```python
from build123d import *

# Parameters (mm, degrees)
F1_DEPTH  = 45
F2_R      = 6
F3_DEPTH  = 10.001
F6_DEPTH  = 6
F7_R      = 10
F8_DEPTH  = 37.5
F10_DEPTH = 3


# Not quite as in the source:
# - a pattern or mirror of a feature is missing from the dataset's text; its kind, count and spacing are read off the source's solid


with BuildPart() as f1:
    # F0 (on Right) → F1 (new body, symmetric)
    with BuildSketch(Plane.YZ):
        Polygon((27.5, -20), (77.5, -20), (77.5, -10), (37.5, -10), (37.5, 0), (-37.5, 0), (-37.5, -10), (-77.5, -10), (-77.5, -20), (-27.5, -20), (-27.5, -10), (27.5, -10), align=None)
    extrude(amount=F1_DEPTH, both=True)

    # F2 (on face) → F3 (cut, through all)
    with BuildSketch(Plane.XY.offset(-10)):
        with Locations((25, -52.5)):
            Circle(F2_R)
        with Locations((-25, -52.5)):
            Circle(F2_R)
        with Locations((-25, 52.5)):
            Circle(F2_R)
        with Locations((25, 52.5)):
            Circle(F2_R)
    extrude(amount=-F3_DEPTH, mode=Mode.SUBTRACT)

    # F5 (on offset) → F6 (join)
    with BuildSketch(Plane(origin=(-8, 0, 0), x_dir=(0, -1, 0), z_dir=(-1, 0, 0))):
        Polygon((-37.5, -10), (-37.5, 0), (-77.5, -10), align=None)
    f6 = extrude(amount=-F6_DEPTH)

    # F6_copies: F6 across plane
    add(f6.mirror(Plane(origin=(0, 0, 0), x_dir=(0, 0, -1), z_dir=(0, -1, 0))))

    # F7 (on Front) → F8 (join, symmetric)
    with BuildSketch(Plane.XZ):
        with BuildLine():
            Line((5, 0), (45, 0))
            Line((45, 0), (45, 35))
            ThreePointArc((45, 35), (25, 55), (5, 35))
            Line((5, 35), (5, 0))
        make_face()
        with Locations((25, 35)):
            Circle(F7_R, mode=Mode.SUBTRACT)
    extrude(amount=F8_DEPTH, both=True)

    # F9 (on Front) → F10 (join, symmetric)
    with BuildSketch(Plane.XZ):
        Polygon((11.7812880283, 50.0088525148), (-45, 0), (5, 0), align=None)
    extrude(amount=F10_DEPTH, both=True)


solid = f1.part
```
Read the model definition and answer for the solid it produces. Units are mm, in the model's axes. A direction names the side the tool comes from. Coordinates: 2 decimals unless noted, no trailing zeros. Loops run counter-clockwise (first coordinate to the right, second up) from the corner with the lowest first, then second, coordinate; pieces in that order, holes last. Notation, with made-up numbers: (73, 39.25) - (115, 39.25) arc R24 ccw to (115, 50.25) - close; hole circle Ø7 at (54, -32.75). An arc over 180 degrees is marked (long way). Answer in a Markdown table with one row per item.
1. Find section C-C, the plane x = 22. Write down the section's boundary in (y, z), then the cut area to 3 significant figures.
Conclusion:
| item | result |
|---|---|
| outline | (-77.5, -20) - (-57.7, -20) - (-57.7, -10) - (-77.5, -10) - close; (-47.3, -20) - (-27.5, -20) - (-27.5, -10) - (27.5, -10) - (27.5, -20) - (47.3, -20) - (47.3, -10) - (37.5, -10) - (37.5, 25.46) - (-37.5, 25.46) - (-37.5, -10) - (-47.3, -10) - close; (-37.5, 44.54) - (37.5, 44.54) - (37.5, 54.77) - (-37.5, 54.77) - close; (57.7, -20) - (77.5, -20) - (77.5, -10) - (57.7, -10) - close |
| area | 4,220 mm² |
2. Find section A-A, the plane z = 38. Write down the section's boundary in (x, y), then the cut area to 3 significant figures.
Conclusion:
| item | result |
|---|---|
| outline | (-1.85, -3) - (5.23, -3) - (5.23, -37.5) - (15.46, -37.5) - (15.46, 37.5) - (5.23, 37.5) - (5.23, 3) - (-1.85, 3) - close; (34.54, -37.5) - (44.77, -37.5) - (44.77, 37.5) - (34.54, 37.5) - close |
| area | 1,580 mm² |
3. Given pin 1 (5 mm diameter, centred on x = 33.5, z = 41, fed in from -Y); pin 2 (10.5 mm diameter, centred on y = -21, z = 16.5, fed in from -X); pin 3 (17 mm diameter, centred on x = -27.5, y = 27, fed in from +Z), each flat-ended and moving along its own axis, determine where each tip first touches the part or whether it passes through.
Conclusion:
| item | result |
|---|---|
| pin 1 | stops at y = -37.5 |
| pin 2 | stops at x = 5 |
| pin 3 | stops at z = 0 |
4. Determine the mould class of faces 4 (the face through (-29.76, 48.85, -14.93)), 5 (the face through (-26, -37.5, -5)), 6 (the face through (-2, -49, -7)) for opening direction Y: +Y half, -Y half, draft (parallel to the pull), parting line (faces both ways), or undercut.
Conclusion:
| item | result |
|---|---|
| face 4 | undercut |
| face 5 | -Y half |
| face 6 | draft |
5. Find section B-B, the plane y = 52.5. Write down the section's boundary in (x, z), then the cut area to 4 significant figures.
Conclusion:
| item | result |
|---|---|
| outline | (-45, -20) - (-31, -20) - (-31, -10) - (-45, -10) - close; (-19, -20) - (19, -20) - (19, -10) - (-2, -10) - (-2, -3.75) - (-8, -3.75) - (-8, -10) - (-19, -10) - close; (31, -20) - (45, -20) - (45, -10) - (31, -10) - close |
| area | 697.5 mm² |
6. Which of the six approach directions +Z, -Z, +X, -X, +Y, -Y give full straight-line access (tool end or side, diameter ignored) to faces 1 (the face through (-20, -20, 0)), 2 (the face through (-8, 49, -7)), 3 (the face through (1, -27.5, -15))?
Conclusion:
| item | result |
|---|---|
| face 1 | +Z, -X, -Y |
| face 2 | +Z, -X, +Y |
| face 3 | -Z, +X, -X |
7. Straight lines are drawn through the part: line 1 (X direction, y = 52, z = -14); line 2 (Y direction, x = -25, z = -14); line 3 (Z direction, x = 25, y = -2). For each, find the intervals that lie inside material, in ascending order.
Conclusion:
| item | result |
|---|---|
| line 1 | x = -45 to -30.98, -19.02 to 19.02, 30.98 to 45 |
| line 2 | y = -77.5 to -58.5, -46.5 to -27.5, 27.5 to 46.5, 58.5 to 77.5 |
| line 3 | z = -10 to 25, 45 to 55 |
8. Find section D-D, the plane y = 29.5. Write down the section's boundary in (x, z), then the cut area to 3 significant figures.
Conclusion:
| item | result |
|---|---|
| outline | (-45, -20) - (45, -20) - (45, 35) arc R20 ccw to (5, 35) - (5, 0) - (-45, 0) - close; hole circle Ø20 at (25, 35) |
| area | 3,510 mm² |
